from build123d import *

# Parameters (mm, degrees)
F1_DEPTH  = 40
F2_R      = 3.25
F3_DEPTH  = 25
F4_R      = 3.25
F4_R_2    = 2
F5_DEPTH  = 25
F6_SIZE   = 5
F7_SIZE   = 5
F8_DEPTH  = 25
F9_W      = 50.789644
F9_H      = 57.590966
F10_DEPTH = 51.1


with BuildPart() as f1:
    # F0 (on Front) → F1 (new body)
    with BuildSketch(Plane.XZ):
        Polygon((0, 50), (0, 0), (50, 0), (50, 5), (5, 5), (5, 50), align=None)
    extrude(amount=F1_DEPTH)

    # F2 (on face) → F3 (cut)
    with BuildSketch(Plane(origin=(0, 0, 0), x_dir=(1, 0, 0), z_dir=(0, 0, -1))):
        with Locations((25, 20)):
            Circle(F2_R)
        with BuildLine():
            ThreePointArc((37.049758, 30.526316), (41, 20), (37.049758, 9.473684))
            ThreePointArc((37.049758, 9.473684), (37.335405, 5.240671), (41.568419, 5.526317))
            ThreePointArc((41.568419, 5.526317), (47, 20.000001), (41.568418, 34.473684))
            ThreePointArc((41.568418, 34.473684), (37.335404, 34.75933), (37.049758, 30.526316))
        make_face()
        with Locations((12.5, 20)):
            Circle(F2_R)
        with Locations((35, 20)):
            Circle(F2_R)
        with BuildLine():
            Line((26.554622, -9.521332), (37.049758, 0))
            ThreePointArc((37.049758, 0), (21.024879, 7.89477), (5, 0))
            Line((5, 0), (26.554622, -9.521332))
        make_face()
        with BuildLine():
            Line((21.024879, 52.316344), (5, 40))
            ThreePointArc((5, 40), (21.024879, 32.105231), (37.049758, 40))
            Line((37.049758, 40), (21.024879, 52.316344))
        make_face()
    extrude(amount=-F3_DEPTH, mode=Mode.SUBTRACT)

    # F4 (on face) → F5 (cut)
    with BuildSketch(Plane(origin=(0, 0, 0), x_dir=(0, -1, 0), z_dir=(-1, 0, 0))):
        with Locations((20, 12.5)):
            Circle(F4_R)
        with Locations((20, 25)):
            Circle(F4_R)
        with Locations((20, 35)):
            Circle(F4_R)
        with BuildLine():
            ThreePointArc((9.473684, 37.049758), (20, 41), (30.526316, 37.049758))
            ThreePointArc((30.526316, 37.049758), (34.75933, 37.335404), (34.473684, 41.568418))
            ThreePointArc((34.473684, 41.568418), (20, 47), (5.526316, 41.568418))
            ThreePointArc((5.526316, 41.568418), (5.24067, 37.335404), (9.473684, 37.049758))
        make_face()
        with Locations((32.5, 12.5)):
            Circle(F4_R_2)
        with Locations((32.5, 25)):
            Circle(F4_R_2)
        with Locations((7.5, 25)):
            Circle(F4_R_2)
        with Locations((7.5, 12.5)):
            Circle(F4_R_2)
    extrude(amount=-F5_DEPTH, mode=Mode.SUBTRACT)

    # F6
    f6_edges = [f1.edges().sort_by_distance(p)[0] for p in [
        (50, -40, 2.5),
    ]]
    chamfer(f6_edges, length=F6_SIZE)

    # F7
    f7_edges = [f1.edges().sort_by_distance(p)[0] for p in [
        (50, 0, 2.5),
    ]]
    chamfer(f7_edges, length=F7_SIZE)

    # F2 (on face) → F8 (cut)
    with BuildSketch(Plane(origin=(0, 0, 0), x_dir=(1, 0, 0), z_dir=(0, 0, -1))):
        with Locations((25, 20)):
            Circle(F2_R)
        with BuildLine():
            ThreePointArc((37.049758, 30.526316), (41, 20), (37.049758, 9.473684))
            ThreePointArc((37.049758, 9.473684), (37.335405, 5.240671), (41.568419, 5.526317))
            ThreePointArc((41.568419, 5.526317), (47, 20.000001), (41.568418, 34.473684))
            ThreePointArc((41.568418, 34.473684), (37.335404, 34.75933), (37.049758, 30.526316))
        make_face()
        with Locations((12.5, 20)):
            Circle(F2_R)
        with Locations((35, 20)):
            Circle(F2_R)
        with BuildLine():
            Line((26.554622, -9.521332), (37.049758, 0))
            ThreePointArc((37.049758, 0), (21.024879, 7.89477), (5, 0))
            Line((5, 0), (26.554622, -9.521332))
        make_face()
        with BuildLine():
            Line((21.024879, 52.316344), (5, 40))
            ThreePointArc((5, 40), (21.024879, 32.105231), (37.049758, 40))
            Line((37.049758, 40), (21.024879, 52.316344))
        make_face()
    extrude(amount=F8_DEPTH, mode=Mode.SUBTRACT)

    # F9 (on face) → F10 (cut)
    with BuildSketch(Plane.XZ.offset(40)):
        with Locations((28.394822, 31.795483)):
            Rectangle(F9_W, F9_H)
    extrude(amount=-F10_DEPTH, mode=Mode.SUBTRACT)


solid = f1.part
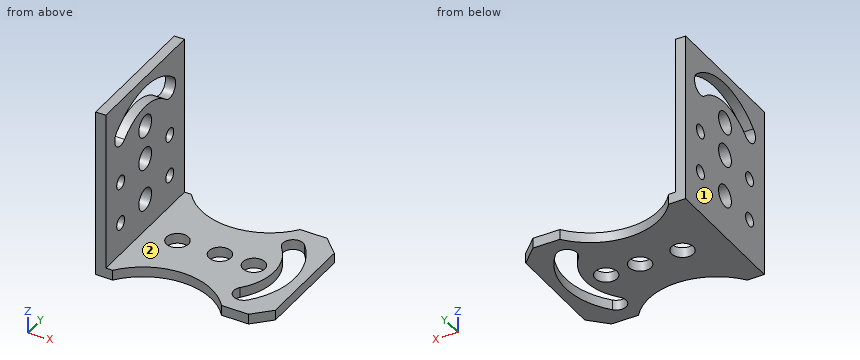
Design review of the part built by this model. Coordinates are the model's own, in mm. Face numbers are marked on the shaded views. A direction names the side the tool comes from. Coordinates: 2 decimals unless noted, no trailing zeros. Loops run counter-clockwise (first coordinate to the right, second up) from the corner with the lowest first, then second, coordinate; pieces in that order, holes last. Notation, with made-up numbers: (43.5, 68.5) - (97.5, 68.5) arc R25 cw to (97.5, 102.5) - close; hole circle Ø4 at (-4, 37). An arc over 180 degrees is marked (long way). Use CSV: the item, a comma, the result in double quotes. Start each with the question number.
1. Add section B-B on z = 35. Give the boundary of the cut face in (x, y), plus the area to 4 significant figures.
2. Clearance check with flat-ended pins moving along their axes: pin 1 (8.5 mm diameter, centred on x = 25, y = -20, fed in from -Z); pin 2 (3 mm diameter, centred on y = -7, z = 37.5, fed in from +X); pin 3 (20 mm diameter, centred on x = 37.5, y = -25, fed in from +Z). State where each tip first meets the part, or that it passes through.
3. For the marked faces 1 and 2, list the 3-axis set-ups (+Z, -Z, +X, -X, +Y, -Y) from which the entire face can be reached by the end or side of a thin tool; tool diameter is ignored.
4. Add section D-D on y = -24.5. Give the boundary of the cut face in (x, z), plus the area to 3 significant figures.
5. To check wall thickness, follow probe 1 along X at (y, z) = (-20, 1.6); probe 2 along X at (y, z) = (-2, 12.5); probe 3 along Y at (x, z) = (2, 12). State the ranges of each line that lie inside material, in increasing order.
6. Add section A-A on x = 25. Give the boundary of the cut face in (y, z), plus the area to 3 significant figures.
7. Add section C-C on z = 12.5. Give the boundary of the cut face in (x, y), plus the area to 3 significant figures.
Resolved:
1,outline,"(0, -40) - (3, -40) - (3, -23.25) - (0, -23.25) - close; (0, -16.75) - (3, -16.75) - (3, 0) - (0, 0) - close"
1,area,"100.5 mm2"
2,pin 1,"z = 0"
2,pin 2,"x = 3"
2,pin 3,"z = 3"
3,face 1,"+Z, -Z, -X, +Y, -Y"
3,face 2,"+Z, +X, +Y, -Y"
4,outline,"(0, 0) - (40.35, 0) - (40.35, 3) - (3, 3) - (3, 40.35) - (0, 40.35) - close; (0, 46.53) - (3, 46.53) - (3, 50) - (0, 50) - close; (46.53, 0) - (50, 0) - (50, 3) - (46.53, 3) - close"
4,area,"254 mm2"
5,probe 1,"0 to 9.25, 15.75 to 21.75, 28.25 to 31.75, 38.25 to 41, 47 to 50"
5,probe 2,"0 to 3"
5,probe 3,"-40 to -34.44, -30.56 to -23.21, -16.79 to -9.44, -5.56 to 0"
6,outline,"(-32.5, 0) - (-23.25, 0) - (-23.25, 3) - (-32.5, 3) - close; (-16.75, 0) - (-7.5, 0) - (-7.5, 3) - (-16.75, 3) - close"
6,area,"55.5 mm2"
7,outline,"(0, -40) - (3, -40) - (3, -34.5) - (0, -34.5) - close; (0, -30.5) - (3, -30.5) - (3, -23.25) - (0, -23.25) - close; (0, -16.75) - (3, -16.75) - (3, -9.5) - (0, -9.5) - close; (0, -5.5) - (3, -5.5) - (3, 0) - (0, 0) - close"
7,area,"76.5 mm2"
